```python
from build123d import *

# Parameters (mm, degrees)
SKETCH1_W           = 66.5
SKETCH1_H           = 68.25
BOSS_EXTRUDE1_DEPTH = 1.5
SKETCH3_R           = 2
SKETCH3_R_2         = 1.5
CUT_EXTRUDE1_DEPTH  = 48.668942982
BOSS_EXTRUDE2_DEPTH = 5


with BuildPart() as part:
    # Sketch1 → Boss-Extrude1 (new body)
    with BuildSketch(Plane(origin=(0, 0, 0), x_dir=(1, 0, 0), z_dir=(0, 1, 0))):
        Rectangle(SKETCH1_W, SKETCH1_H)
    extrude(amount=BOSS_EXTRUDE1_DEPTH)

    # Sketch3 → Cut-Extrude1 (cut, through all)
    with BuildSketch(Plane(origin=(0, 1.5, 0), x_dir=(1, 0, 0), z_dir=(0, 1, 0))):
        with Locations(Location((-30, -28.317585536, 0), (0, 0, 270))):
            Circle(SKETCH3_R)
        with Locations(Location((30, -28.317585536, 0), (0, 0, 270))):
            Circle(SKETCH3_R)
        with Locations(Location((30, 25.682414464, 0), (0, 0, 270))):
            Circle(SKETCH3_R)
        with Locations(Location((-30, 25.682414464, 0), (0, 0, 270))):
            Circle(SKETCH3_R)
        with Locations(Location((30, 7.682414464, 0), (0, 0, 270))):
            Circle(SKETCH3_R_2)
        with Locations(Location((30, -10.317585536, 0), (0, 0, 270))):
            Circle(SKETCH3_R_2)
        with Locations(Location((-30, -10.317585536, 0), (0, 0, 90))):
            Circle(SKETCH3_R_2)
        with Locations(Location((-30, 7.682414464, 0), (0, 0, 90))):
            Circle(SKETCH3_R_2)
    extrude(amount=-CUT_EXTRUDE1_DEPTH, mode=Mode.SUBTRACT)

    # Sketch5 → Boss-Extrude2 (add)
    # profile 1 of 5: a face of its own
    with BuildSketch(Plane(origin=(0, 1.5, 0), x_dir=(1, 0, 0), z_dir=(0, 1, 0))):
        Polygon((-14.006270714, 21.19159661), (-11.506270714, 21.19159661), (-10.006270714, 19.89159661), (-10.006270714, 10.69159661), (-14.006270714, 10.69159661), align=None)
        Polygon((-10.406270714, 19.708945057), (-10.406270714, 12.008945057), (-11.656270714, 11.09159661), (-13.606270714, 11.09159661), (-13.606270714, 20.79159661), (-11.655484044, 20.79159661), align=None, mode=Mode.SUBTRACT)
    # profile 2 of 5: a face of its own
    with BuildSketch(Plane(origin=(0, 1.5, 0), x_dir=(1, 0, 0), z_dir=(0, 1, 0))):
        Polygon((-9.006270714, 21.19159661), (-6.506270714, 21.19159661), (-5.006270714, 19.89159661), (-5.006270714, 10.69159661), (-9.006270714, 10.69159661), align=None)
        Polygon((-5.406270714, 19.708945057), (-5.406270714, 12.008945057), (-6.656270714, 11.09159661), (-8.606270714, 11.09159661), (-8.606270714, 20.79159661), (-6.655484044, 20.79159661), align=None, mode=Mode.SUBTRACT)
    # profile 3 of 5: a face of its own
    with BuildSketch(Plane(origin=(0, 1.5, 0), x_dir=(1, 0, 0), z_dir=(0, 1, 0))):
        Polygon((-4.006270714, 21.19159661), (-1.506270714, 21.19159661), (-0.006270714, 19.89159661), (-0.006270714, 10.69159661), (-4.006270714, 10.69159661), align=None)
        Polygon((-0.406270714, 19.708945057), (-0.406270714, 12.008945057), (-1.656270714, 11.09159661), (-3.606270714, 11.09159661), (-3.606270714, 20.79159661), (-1.655484044, 20.79159661), align=None, mode=Mode.SUBTRACT)
    # profile 4 of 5: a face of its own
    with BuildSketch(Plane(origin=(0, 1.5, 0), x_dir=(1, 0, 0), z_dir=(0, 1, 0))):
        Polygon((0.993729286, 21.19159661), (3.493729286, 21.19159661), (4.993729286, 19.89159661), (4.993729286, 10.69159661), (0.993729286, 10.69159661), align=None)
        Polygon((4.593729286, 19.708945057), (4.593729286, 12.008945057), (3.343729286, 11.09159661), (1.393729286, 11.09159661), (1.393729286, 20.79159661), (3.344515956, 20.79159661), align=None, mode=Mode.SUBTRACT)
    # profile 5 of 5: a face of its own
    with BuildSketch(Plane(origin=(0, 1.5, 0), x_dir=(1, 0, 0), z_dir=(0, 1, 0))):
        Polygon((5.993729286, 21.19159661), (8.493729286, 21.19159661), (9.993729286, 19.89159661), (9.993729286, 10.69159661), (5.993729286, 10.69159661), align=None)
        Polygon((9.593729286, 19.708945057), (9.593729286, 12.008945057), (8.343729286, 11.09159661), (6.393729286, 11.09159661), (6.393729286, 20.79159661), (8.344515956, 20.79159661), align=None, mode=Mode.SUBTRACT)
    extrude(amount=BOSS_EXTRUDE2_DEPTH)


solid = part.part
```
Read the model definition and answer for the solid it produces. Units are mm, in the model's axes. A direction names the side the tool comes from. Round coordinates to 2 decimals unless told otherwise and drop trailing zeros. Write each loop counter-clockwise with the first axis right and the second up, starting at its lowest first coordinate (ties: lowest second). Pieces come first, ordered by that corner, then holes. Notation, with made-up numbers: (50.5, 44.5) - (62.5, 44.5) arc R4 ccw to (62.5, 51.5) - close; hole circle Ø11 at (14, -19.75). An arc over 180 degrees is marked (long way). One line per item, written item: value.
Q1. Each of these flat-tipped pins is pushed along its axis until it touches: P1, Ø1.5, axis at y = 4.5, z = -13.5, coming from the +X side; P2, Ø2, axis at x = -2.5, y = 5, coming from the +Z side; P3, Ø2, axis at x = -12.5, y = 5, coming from the -Z side. Where does it stop, or does it pass through?
The answers:
P1: stops at x = 9.99
P2: stops at z = -10.69
P3: stops at z = -21.19
Q2. Find section C-C (y = 2.5). Count the separate pieces of the cut face and the enclosed holes in it, and give its area (3 significant figures).
The answers:
separate pieces: 5
enclosed holes: 5
area: 56.2 mm2
Q3. Which of the six approach directions +Z, -Z, +X, -X, +Y, -Y give full straight-line access (tool end or side, diameter ignored) to faces 1 (the flat face through (-5.767, 3.965, -20.551)), 2 (the flat face through (-7, 4, -10.692)), 3 (the flat face through (5.994, 4, -16)), 4 (the flat face through (-7, 1.5, -16)), 5 (the flat face through (9.233, 3.965, -20.551))?
The answers:
face 1: -Z, +Y
face 2: +Z, +X, -X, +Y
face 3: +Z, -Z, +Y
face 4: +Y
face 5: -Z, +X, +Y
Q4. Find section D-D (x = 19). Determine the outline of the cut face in (y, z) (3 decimals).
The answers:
outline: (0, -34.125) - (1.5, -34.125) - (1.5, 34.125) - (0, 34.125) - close
Q5. Find section A-A (x = -30). Determine the outline of the cut face in (y, z) (3 decimals), and give its area (3 significant figures).
The answers:
outline: (0, -34.125) - (1.5, -34.125) - (1.5, -27.682) - (0, -27.682) - close; (0, -23.682) - (1.5, -23.682) - (1.5, -9.182) - (0, -9.182) - close; (0, -6.182) - (1.5, -6.182) - (1.5, 8.818) - (0, 8.818) - close; (0, 11.818) - (1.5, 11.818) - (1.5, 26.318) - (0, 26.318) - close; (0, 30.318) - (1.5, 30.318) - (1.5, 34.125) - (0, 34.125) - close
area: 81.4 mm2
Q6. Straight lines are drawn through the part: line 1 (Y direction, x = -4, z = 31.5); line 2 (Z direction, x = -8, y = 4.25); line 3 (Z direction, x = 9.5, y = 5). For each, find the intervals that lie inside material, in ascending order. Write a range as from..to.
The answers:
line 1: y = 0..1.5
line 2: z = -21.19..-20.79, -11.09..-10.69
line 3: z = -20.32..-19.79, -11.94..-10.69
Q7. Find section B-B (z = -7.5). Determine the outline of the cut face in (x, y).
The answers:
outline: (-33.25, 0) - (-31.49, 0) - (-31.49, 1.5) - (-33.25, 1.5) - close; (-28.51, 0) - (28.51, 0) - (28.51, 1.5) - (-28.51, 1.5) - close; (31.49, 0) - (33.25, 0) - (33.25, 1.5) - (31.49, 1.5) - close
Q8. For a pull along Z with two mould halves and no side action, classify faces 6 (the flat face through (0.994, 4, -16)), 7 (the flat face through (-8, 4, -20.792)), 8 (the flat face through (-2, 4, -10.692)), 9 (the flat face through (0, 1, -34.125)) as pulls with the +Z half, pulls with the -Z half, needs draft (parallel to the pull), parting line crosses it, or undercut.
The answers:
face 6: needs draft
face 7: undercut
face 8: pulls with the +Z half
face 9: pulls with the -Z half
